Autodesk Inventor part; units mm, degrees
ref_plane "YZ Plane" through (0, 0, 0) normal (1, 0, 0) x (0, 1, 0)
ref_plane "XZ Plane" through (0, 0, 0) normal (0, 1, 0) x (-1, 0, 0)
ref_plane "XY Plane" through (0, 0, 0) normal (0, 0, 1) x (1, 0, 0)
sketch "Эскиз1" plane through (0, 0, 0) normal (0, 0, 1) x (1, 0, 0)
  circle A0 centre (0, 0) radius 18
  circle A1 centre (0, 0) radius 20
  dimension "d0" = 36
  dimension "d1" = 40
extrude "Выдавливание1" add sketch "Эскиз1" along normal blind 2
sketch "Эскиз2" plane through (0, 0, 2) normal (0, 0, 1) x (1, 0, 0)
  circle A0 centre (0, 0) radius 20
  circle A1 centre (0, 0) radius 16.5
  dimension "d4" = 33
extrude "Выдавливание2" add sketch "Эскиз2" along normal blind 1.25
mirror "Зеркальное отражение1" about plane through (0, 0, 0) normal (0, 0, -1)
properties part number "Шина колеса D40"
Can you work these out from the model? Positions are in its coordinate system, mm. A direction names the side the tool comes from. Coordinates: 2 decimals unless noted, no trailing zeros. Loops run counter-clockwise (first coordinate to the right, second up) from the corner with the lowest first, then second, coordinate; pieces in that order, holes last. Notation, with made-up numbers: (56.25, -36) - (60.25, -36) arc R17 ccw to (60.25, -7) - close; hole circle Ø7 at (88, 83.5). An arc over 180 degrees is marked (long way). Use a Markdown table: item, result.
Item 1: I want a section at A-A on y = 0. Please give me the cut outline in (x, z).
Numbers:
| item | result |
|---|---|
| outline | (-20, -3.25) - (-16.5, -3.25) - (-16.5, -2) - (-18, -2) - (-18, 2) - (-16.5, 2) - (-16.5, 3.25) - (-20, 3.25) - close; (16.5, -3.25) - (20, -3.25) - (20, 3.25) - (16.5, 3.25) - (16.5, 2) - (18, 2) - (18, -2) - (16.5, -2) - close |
Item 2: We'd pull the mould along Y, two halves only. Please class faces 3 (the face through (2.9, 16.4, 3.25)), 4 (the face through (15.24, 6.32, 2.62)), 5 (the face through (-4.336, 19.524, -0.046)): released by +Y, released by -Y, zero draft, split by the parting line, or undercut.
Numbers:
| item | result |
|---|---|
| face 3 | zero draft |
| face 4 | undercut |
| face 5 | split by the parting line |
Item 3: I want a section at C-C on z = -0.5. Please give me the cut outline in (x, y), and give its area (3 significant figures).
Numbers:
| item | result |
|---|---|
| outline | circle Ø40 at (0, 0); hole circle Ø36 at (0, 0) |
| area | 239 mm2 |
Item 4: If I drill on probe 1 along Y at (x, z) = (0, 2.85); probe 2 along X at (y, z) = (0.5, 1); probe 3 along Y at (x, z) = (11, -1.75), over which ranges is the centre line in solid material (lowest first)? Write a range as from..to.
Numbers:
| item | result |
|---|---|
| probe 1 | y = -20..-16.5, 16.5..20 |
| probe 2 | x = -19.99..-17.99, 17.99..19.99 |
| probe 3 | y = -16.7..-14.25, 14.25..16.7 |
Item 5: For faces 1 (the face through (-2.9, 16.4, -3.25)), 2 (the face through (8, -15, 2)), which set-ups out of +Z, -Z, +X, -X, +Y, -Y let a thin tool reach every point of the face, with its end or its side?
Numbers:
| item | result |
|---|---|
| face 1 | -Z, +X, -X, +Y, -Y |
| face 2 | none |
Item 6: Will these pins go through, and if not, where does the flat tip stop? pin 1 (18 mm diameter, centred on x = 4.5, y = 7, fed in from -Z); pin 2 (3 mm diameter, centred on y = -5.5, z = -2, fed in from +X); pin 3 (1.5 mm diameter, centred on x = 4.5, z = 1, fed in from -Y).
Numbers:
| item | result |
|---|---|
| pin 1 | stops at z = -3.25 |
| pin 2 | stops at x = 19.6 |
| pin 3 | stops at y = -19.65 |
